Can you work these out from the model? Positions are in its coordinate system, mm. A direction names the side the tool comes from. Give positions to 0.01 mm unless a question says otherwise; leave off trailing zeros. Order: outer loops, then holes, each group sorted by start corner. A loop starts at its lowest first (then second) coordinate and runs counter-clockwise, first axis right, second up. Notation, with made-up numbers: (-29, -25.5) - (-4, -25.5) arc R36 cw to (-4, 9.5) - close; hole circle Ø11 at (26, -25). An arc over 180 degrees is marked (long way). Use one line per item in the form item = value. Start each with the question number.
1) Suppose I cut it at C-C, the plane y = 0. Write out the boundary of the cut face in (x, z).
2) Suppose I cut it at A-A, the plane x = 0. Write out the boundary of the cut face in (y, z), and give its area (3 significant figures).
3) Suppose I cut it at D-D, the plane z = 16.25. Write out the boundary of the cut face in (x, y), and give its area (3 significant figures).
4) Which directions (+Z, -Z, +X, -X, +Y, -Y) give clear straight access to the entire face, cutting with the end or side of a thin tool? Please do faces 4 (the flat face through (0, 18.75, 11)), 5 (the cylindrical face through (5.002, -5.834, 15.544)).
5) For pin 1 (4 mm diameter, centred on x = -5, y = -3.5, fed in from +Z); pin 2 (3 mm diameter, centred on y = -8, z = 18.5, fed in from -X), each with a flat end and sliding along its axis, tell me the tip position at first contact or that it passes through.
6) Suppose I cut it at B-B, the plane y = 14.65. Write out the boundary of the cut face in (x, z), and give its area (3 significant figures).
7) We'd pull the mould along Y, two halves only. Please class faces 1 (the flat face through (-15.56, 0, 11)), 2 (the flat face through (0, -18.75, 11)), 3 (the cylindrical face through (-0.89, -16.04, 10.79)): released by +Y, released by -Y, zero draft, split by the parting line, or undercut.
8) Please list where these lines run through material, in increasing order: probe 1 along Y at (x, z) = (0, 10.7); probe 2 along X at (y, z) = (-14.65, 10.5); probe 3 along Z at (x, y) = (-6, -14.5).
```python
from build123d import *

# Parameters (mm, degrees)
SKETCH018_W             = 31.12
SKETCH018_H             = 37.5
PAD010_DEPTH            = 1.6
SKETCH019_R             = 1.65
POCKET006_DEPTH         = 99.115397
SKETCH032_R             = 3.25
PAD018_DEPTH            = 8
BODY003_PLACEMENT_ANGLE = 180


with BuildPart() as part:
    # Sketch018 → Pad010 (new body)
    with BuildSketch(Plane.XY):
        Rectangle(SKETCH018_W, SKETCH018_H)
    extrude(amount=PAD010_DEPTH)

    # Sketch019 (on Face5 of Pad010) → Pocket006 (cut, through all)
    with BuildSketch(Plane(origin=(0, 0, 0), x_dir=(1, 0, 0), z_dir=(0, 0, -1))):
        with Locations((0, 14.65)):
            Circle(SKETCH019_R)
    pocket006 = extrude(amount=-POCKET006_DEPTH, mode=Mode.SUBTRACT)

    # Mirrored008: Pocket006 across Sketch019 H_Axis
    add(pocket006.mirror(Plane(origin=(0, 0, 0), x_dir=(0, 0, -1), z_dir=(0, -1, 0))), mode=Mode.SUBTRACT)

    # Sketch032 (on Face5 of Mirrored008) → Pad018 (join)
    with BuildSketch(Plane.XY.offset(1.6)):
        with Locations((-4.296995, 9.00655)):
            Circle(SKETCH032_R)
    extrude(amount=PAD018_DEPTH)


with BuildPart() as part_1:
    # Body003 placement: moved
    add(part.part.moved(Location((0, 0, 10))).rotate(Axis((0, 0, 10), (0, 0, 1)), BODY003_PLACEMENT_ANGLE))


solid = part_1.part
```
Result sheet:
q1.outline = (-15.56, 10) - (15.56, 10) - (15.56, 11.6) - (-15.56, 11.6) - close
q2.outline = (-18.75, 10) - (-16.3, 10) - (-16.3, 11.6) - (-18.75, 11.6) - close; (-13, 10) - (13, 10) - (13, 11.6) - (-13, 11.6) - close; (16.3, 10) - (18.75, 10) - (18.75, 11.6) - (16.3, 11.6) - close
q2.area = 49.4 mm²
q3.outline = circle Ø6.5 at (4.3, -9.01)
q3.area = 33.2 mm²
q4.face_4 = +Z, -Z, +X, -X, +Y
q4.face_5 = +Z
q5.pin_1 = 11.6
q5.pin_2 = 1.05
q6.outline = (-15.56, 10) - (-1.65, 10) - (-1.65, 11.6) - (-15.56, 11.6) - close; (1.65, 10) - (15.56, 10) - (15.56, 11.6) - (1.65, 11.6) - close
q6.area = 44.5 mm²
q7.face_1 = zero draft
q7.face_2 = released by -Y
q7.face_3 = undercut
q8.probe_1 = -18.75 to -16.3, -13 to 13, 16.3 to 18.75
q8.probe_2 = -15.56 to -1.65, 1.65 to 15.56
q8.probe_3 = 10 to 11.6
